Verification items for the finished model (mm, model axes). Give positions to 0.01 mm unless a question says otherwise; leave off trailing zeros. Order: outer loops, then holes, each group sorted by start corner. A loop starts at its lowest first (then second) coordinate and runs counter-clockwise, first axis right, second up.
from build123d import *

# Parameters (mm, degrees)
F0_W     = 831.85
F0_H     = 50.8
F1_DEPTH = 20.6375
F2_W     = 12.7
F2_H     = 6.35
F3_DEPTH = 831.85
F4_W     = 12.7
F4_H     = 6.35
F5_DEPTH = 50.801


with BuildPart() as f1:
    # F0 (on Top) → F1 (new body)
    with BuildSketch(Plane.XY):
        with Locations((415.925, 25.4)):
            Rectangle(F0_W, F0_H)
    extrude(amount=F1_DEPTH)

    # F2 (on Right) → F3 (cut, through all)
    with BuildSketch(Plane.YZ):
        with Locations((6.35, 9.525)):
            Rectangle(F2_W, F2_H)
    extrude(amount=F3_DEPTH, mode=Mode.SUBTRACT)

    # F4 (on Front) → F5 (cut, through all)
    with BuildSketch(Plane.XZ):
        with Locations((6.35, 9.525)):
            Rectangle(F4_W, F4_H)
        with Locations((825.5, 9.525)):
            Rectangle(F4_W, F4_H)
    extrude(amount=-F5_DEPTH, mode=Mode.SUBTRACT)


solid = f1.part
(1) Scan lines: line 1 (Z direction, x = 238, y = 12.5); line 2 (Y direction, x = 163.5, z = 9); line 3 (X direction, y = 49, z = 9.75). Record each from-to range of solid material in increasing order.
Solved:
line 1: z = 0 to 6.35, 12.7 to 20.64
line 2: y = 12.7 to 50.8
line 3: x = 12.7 to 819.15
(2) Release check for a two-part mould opening along Z. For faces 1 (the flat face through (410, 50.8, 10)), 2 (the flat face through (414, 5, 6.35)), 3 (the flat face through (410, 26, 20.638)) record: pulls with the +Z half, pulls with the -Z half, needs draft (parallel to the pull), parting line crosses it, or undercut.
Solved:
face 1: needs draft
face 2: undercut
face 3: pulls with the +Z half
(3) Section check A-A, the plane x = 589. Enter the section's corners in (y, z), then the cut area to 3 significant figures.
Solved:
outline: (0, 0) - (50.8, 0) - (50.8, 20.64) - (0, 20.64) - (0, 12.7) - (12.7, 12.7) - (12.7, 6.35) - (0, 6.35) - close
area: 968 mm2
(4) Go/stop test with flat-tipped pins: pin 1 (4 mm diameter, centred on x = 690.5, z = 9.5, fed in from -Y); pin 2 (1 mm diameter, centred on y = 39, z = 10, fed in from -X); pin 3 (1.9 mm diameter, centred on y = 35, z = 9.5, fed in from +X). Record where each tip stops, or that it passes through.
Solved:
pin 1: stops at y = 12.7
pin 2: stops at x = 12.7
pin 3: stops at x = 819.15
